For this review, take the finished solid that the model builds, in its own axes (mm). Face numbers are marked on the shaded views. Give positions to 0.01 mm unless a question says otherwise; leave off trailing zeros. Order: outer loops, then holes, each group sorted by start corner. A loop starts at its lowest first (then second) coordinate and runs counter-clockwise, first axis right, second up. Notation, with made-up numbers: M -4,3.5 L 40,3.5 A34 cw 40,42.5 Z; hole C 82.25,7.25 d7. An arc over 180 degrees is marked long. Answer as CSV lines item,"result". Start each with the question number.
1. For line 1 along Y through (x, z) = (-25.4, 2.5); line 2 along X through (y, z) = (-6.5, 1); line 3 along Y through (x, z) = (25.4, 3.5), list the stretches that pass through material, from the lowest coordinate up.
2. We need section A-A, the plane x = 33. Give the boundary of the cut face in (y, z), and give its area (3 significant figures).
3. Mouldability with a two-part tool opening along X and no side actions: class the marked faces 1, 2 and 3 as pulls with the +X half, pulls with the -X half, needs draft (parallel to the pull), parting line crosses it, or undercut.
4. Clearance check with flat-ended pins moving along their axes: P1, Ø6, axis at x = 28, y = -2.5, coming from the +Z side; P2, Ø1, axis at x = -22, z = 1.5, coming from the +Y side; P3, Ø1.5, axis at y = -18.5, z = 5, coming from the +X side. State where each tip first meets the part, or that it passes through.
5. We need section B-B, the plane y = -5. State how many separate pieces and enclosed holes the cut face has, and give its area (3 significant figures).
from build123d import *

# Parameters (mm, degrees)
F0_R     = 10.9982
F1_DEPTH = 6.35


with BuildPart() as f1:
    # F0 (on Top) → F1 (new body)
    with BuildSketch(Plane.XY):
        with BuildLine():
            add(Edge.make_bspline(
                [(0, -13.97), (5.7787014373, -13.97), (13.1291277882, -20.32), (18.7630429864, -26.67), (25.4, -26.67)],
                knots=[0, 0, 0, 0, 0.5, 1, 1, 1, 1], degree=3))
            ThreePointArc((25.4, -26.67), (39.37, -12.7), (25.4, 1.27))
            add(Edge.make_bspline(
                [(0, 13.97), (6.853028044, 13.97), (12.6391638998, 7.6416874466), (18.8445616513, 1.27), (25.4, 1.27)],
                knots=[0, 0, 0, 0, 0.500853834, 1, 1, 1, 1], degree=3))
            add(Edge.make_bspline(
                [(-25.4, 26.67), (-17.5831354201, 26.67), (-13.6102278083, 17.9003816405), (-6.4407057817, 14.2221620935), (0, 13.97)],
                knots=[0, 0, 0, 0, 0.5099402335, 1, 1, 1, 1], degree=3))
            ThreePointArc((-25.4, 26.67), (-39.37, 12.7), (-25.4, -1.27))
            add(Edge.make_bspline(
                [(-25.4, -1.27), (-17.5831354201, -1.27), (-13.269427077, -7.7050659785), (-6.678010426, -13.799868043), (0, -13.97)],
                knots=[0, 0, 0, 0, 0.5, 1, 1, 1, 1], degree=3))
        make_face()
        Circle(F0_R, mode=Mode.SUBTRACT)
        with Locations((25.4, -12.7)):
            Circle(F0_R, mode=Mode.SUBTRACT)
        with Locations((-25.4, 12.7)):
            Circle(F0_R, mode=Mode.SUBTRACT)
    extrude(amount=F1_DEPTH)


solid = f1.part
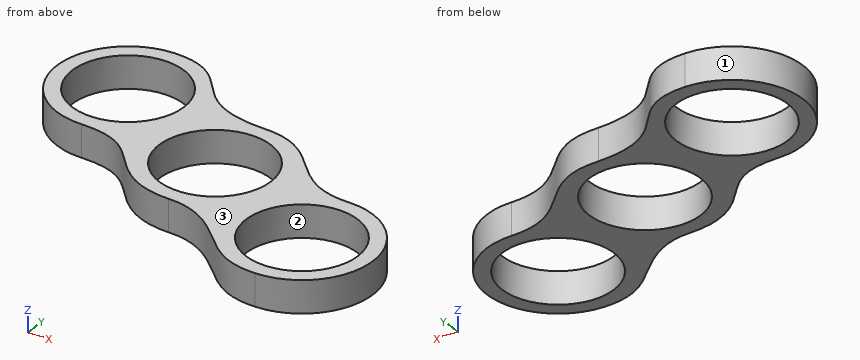
Result set:
1,line 1,"-1.27 to 1.7, 23.7 to 26.67"
1,line 2,"-13.66 to -8.87, 8.87 to 16.32, 34.48 to 37.92"
1,line 3,"-26.67 to -23.7, -1.7 to 1.27"
2,outline,"M -24.42,0 L -20.65,0 L -20.65,6.35 L -24.42,6.35 Z; M -4.75,0 L -0.98,0 L -0.98,6.35 L -4.75,6.35 Z"
2,area,"47.9 mm2"
3,face 1,"pulls with the -X half"
3,face 2,"undercut"
3,face 3,"needs draft"
4,P1,"z = 6.35"
4,P2,"y = 26.43"
4,P3,"x = 38.43"
5,separate pieces,"3"
5,enclosed holes,"0"
5,area,"107 mm2"
